Could you check a few things on this model? Use its own coordinates, in mm. Face numbers are marked on the shaded views. A direction names the side the tool comes from. Give positions to 0.01 mm unless a question says otherwise; leave off trailing zeros. Write each loop counter-clockwise with the first axis right and the second up, starting at its lowest first coordinate (ties: lowest second). Pieces come first, ordered by that corner, then holes. Notation, with made-up numbers: (39.25, 14.25) -> (89.25, 14.25) arc R6 ccw to (89.25, 21.25) -> close; hole circle Ø11 at (7.25, 69). An arc over 180 degrees is marked (long way). One line per question, with ' | ' between items.
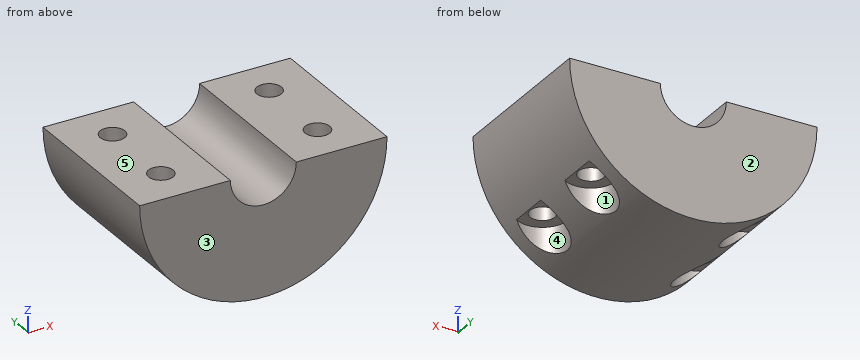
Solid Edge part; units mm, degrees
sketch "Sketch1" plane through (0, 0, 0) normal (0, -1, 0) x (1, 0, 0)
  line L0 (4, 0) -> (15, 0)
  line L1 (-15, 0) -> (-4, 0)
  arc A0 (-4, 0) -> (4, 0) centre (0, 0) ccw
  arc A1 (15, 0) -> (-15, 0) centre (0, 0) cw
extrude "Protrusion1" add sketch "Sketch1" against normal blind 30
sketch "Sketch2" plane through (9.5, 15, 0) normal (0, 0, 1) x (0, 1, 0)
  line L0 (-10, -5.5) -> (10, -5.5)
  line L1 (10, -5.5) -> (10, 24.5)
  line L2 (10, 24.5) -> (-10, 24.5)
  line L3 (-10, 24.5) -> (-10, -5.5)
  line L4 (20, -7.2229) -> (-20, -7.2229)
  line L5 (-20, -7.2229) -> (-20, 26.2229)
  line L6 (-20, 26.2229) -> (20, 26.2229)
  line L7 (20, 26.2229) -> (20, -7.2229)
extrude "ExtrudedCutout_3" cut sketch "Sketch2" against normal blind 40
sketch "Sketch3" plane through (-9.5, 15, 0) normal (0, 0, 1) x (1, 0, 0)
  circle A0 centre (0, 5) radius 1.5
  circle A1 centre (0, -5) radius 1.5
  circle A2 centre (19, -5) radius 1.5
  circle A3 centre (19, 5) radius 1.5
extrude "ExtrudedCutout_4" cut sketch "Sketch3" against normal blind 20
sketch "Sketch4" plane through (9.5, 15, -20) normal (0, 0, 1) x (1, 0, 0)
  circle A0 centre (0, 5) radius 3
  circle A1 centre (0, -5) radius 3
  circle A2 centre (-19, -5) radius 3
  circle A3 centre (-19, 5) radius 3
extrude "ExtrudedCutout_5" cut sketch "Sketch4" along normal blind 10
Q1. Imagine slicing it at C-C on x = 9. Please give me the cut outline in (y, z).
Answer below:
outline: (5, -12) -> (7.04, -12) -> (7.04, -10) -> (8.59, -10) -> (8.59, 0) -> (5, 0) -> close; (11.41, -10) -> (12.96, -10) -> (12.96, -12) -> (17.04, -12) -> (17.04, -10) -> (18.59, -10) -> (18.59, 0) -> (11.41, 0) -> close; (21.41, -10) -> (22.96, -10) -> (22.96, -12) -> (25, -12) -> (25, 0) -> (21.41, 0) -> close
Q2. Imagine slicing it at A-A on z = -3.5. Please give me the cut outline in (x, y).
Answer below:
outline: (-14.59, 5) -> (-1.94, 5) -> (-1.94, 25) -> (-14.59, 25) -> close; (1.94, 5) -> (14.59, 5) -> (14.59, 25) -> (1.94, 25) -> close; hole circle Ø3 at (-9.5, 10); hole circle Ø3 at (-9.5, 20); hole circle Ø3 at (9.5, 10); hole circle Ø3 at (9.5, 20)
Q3. On a 3-axis mill with a long thin cutter (end or side, diameter ignored), from which of +Z, -Z, +X, -X, +Y, -Y can I reach the whole of each face in a straight line? I mean the marked faces 1 and 2. Say none if no direction works.
Answer below:
face 1: -Z | face 2: +Z, -Z, +X, -X, +Y
Q4. Imagine slicing it at B-B on y = 10. Please give me the cut outline in (x, z), and give its area (3 significant figures).
Answer below:
outline: (-15, 0) arc R15 ccw to (-11.18, -10) -> (-11, -10) -> (-11, 0) -> close; (-8, -10) -> (-6.5, -10) -> (-6.5, -13.52) arc R15 ccw to (6.5, -13.52) -> (6.5, -10) -> (8, -10) -> (8, 0) -> (4, 0) arc R4 cw to (-4, 0) -> (-8, 0) -> close; (11, -10) -> (11.18, -10) arc R15 ccw to (15, 0) -> (11, 0) -> close | area: 250 mm^2
Q5. Will these pins go through, and if not, where does the flat tip stop? pin 1 (2.5 mm diameter, centred on x = 7.5, y = 19, fed in from -Z); pin 2 (4 mm diameter, centred on x = -9.5, y = 20, fed in from -Z); pin 3 (2.5 mm diameter, centred on x = -8, y = 11.5, fed in from -Z).
Answer below:
pin 1: stops at z = -13.64 | pin 2: stops at z = -10 | pin 3: stops at z = -13.4
Q6. Imagine slicing it at D-D on z = -5.75. Please give me the cut outline in (x, y).
Answer below:
outline: (-13.85, 5) -> (13.85, 5) -> (13.85, 25) -> (-13.85, 25) -> close; hole circle Ø3 at (-9.5, 10); hole circle Ø3 at (-9.5, 20); hole circle Ø3 at (9.5, 10); hole circle Ø3 at (9.5, 20)
Q7. If we mould it in two halves opening along Y, with no side actions, what happens to the marked faces 3, 4 and 5? For each: +Y half, -Y half, draft (parallel to the pull), parting line (faces both ways), or undercut.
Answer below:
face 3: -Y half | face 4: undercut | face 5: draft
Q8. If I drill on line 1 along Y through (x, z) = (-9.5, -10.9); line 2 along Y through (x, z) = (9.5, -5.75); line 3 along X through (y, z) = (11, -5.75), over which ranges is the centre line in solid material (lowest first)?
Answer below:
line 1: y = 5 to 7, 13 to 17, 23 to 25 | line 2: y = 5 to 8.5, 11.5 to 18.5, 21.5 to 25 | line 3: x = -13.85 to -10.62, -8.38 to 8.38, 10.62 to 13.85
